Print and shaded views of the part. All mm, measured from the part's lowest x, y and z. A direction names the side the tool comes from. Coordinates: 2 decimals unless noted, no trailing zeros. Order: outer loops, then holes, each group sorted by start corner. A loop starts at its lowest first (then second) coordinate and runs counter-clockwise, first axis right, second up. Notation, with made-up numbers: M -7.75,-35 L 38.25,-35 A21 ccw 38.25,-20 Z; hole C 47,2 d2. An arc over 180 degrees is marked long. Use a Markdown table: item, result. Add a question column.
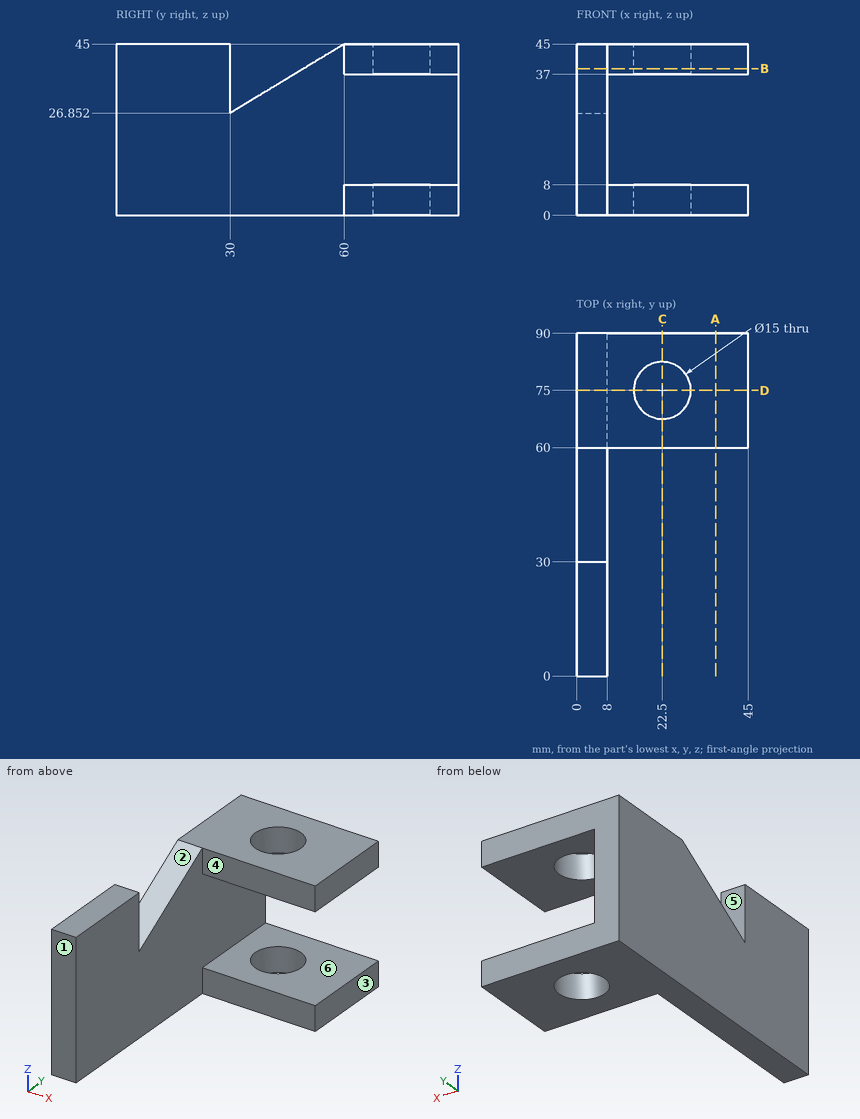
(1) Drop flat-ended pins along their axis: P1, Ø15, axis at x = 21, y = 74.5, coming from the -Z side; P2, Ø8, axis at x = 24.5, z = 15.5, coming from the -Y side; P3, Ø1, axis at y = 52, z = 19.5, coming from the +X side; P4, Ø6.5, axis at x = 34.5, z = 42, coming from the -Y side. Give the stop position or say it passes through.
(2) Drill centre lines: line 1 along Y through (x, z) = (22.5, 40.75); line 2 along Z through (x, y) = (33, 84); line 3 along Y through (x, z) = (39.5, 6). Where is each one in solid material? Low to high. Write a range as from..to.
(3) Mould opens along Y. For the marked faces 1, 2 and 3 say: released by +Y, released by -Y, zero draft, split by the parting line, or undercut.
(4) Slice it at C-C on x = 22.5. Give the cut face in (y, z).
(5) Which spindle directions (+Z, -Z, +X, -X, +Y, -Y) get a long thin tool onto all of the face, cutting with end or side? Do the marked faces 4, 5 and 6. Say none if no direction does.
(6) Slice it at A-A on x = 36.5. Give the cut face in (y, z).
(7) Slice it at B-B on z = 38.5. Give the cut face in (x, y) (3 decimals), and give its area (3 significant figures).
(8) Slice it at D-D on y = 75. Give the cut face in (x, z).
Solutions:
| question | item | result |
|---|---|---|
| 1 | P1 | z = 0 |
| 1 | P2 | through |
| 1 | P3 | x = 8 |
| 1 | P4 | y = 60 |
| 2 | line 1 | 60..67.5, 82.5..90 |
| 2 | line 2 | 0..8, 37..45 |
| 2 | line 3 | 60..90 |
| 3 | face 1 | released by -Y |
| 3 | face 2 | undercut |
| 3 | face 3 | zero draft |
| 4 | outline | M 60,0 L 67.5,0 L 67.5,8 L 60,8 Z; M 60,37 L 67.5,37 L 67.5,45 L 60,45 Z; M 82.5,0 L 90,0 L 90,8 L 82.5,8 Z; M 82.5,37 L 90,37 L 90,45 L 82.5,45 Z |
| 5 | face 4 | +Z, -Z, +X, -Y |
| 5 | face 5 | +Z, +X, -X |
| 5 | face 6 | +X, +Y, -Y |
| 6 | outline | M 60,0 L 90,0 L 90,8 L 60,8 Z; M 60,37 L 90,37 L 90,45 L 60,45 Z |
| 7 | outline | M 0,0 L 8,0 L 8,30 L 0,30 Z; M 0,49.255 L 8,49.255 L 8,60 L 45,60 L 45,90 L 0,90 Z; hole C 22.5,75 d15 |
| 7 | area | 1,500 mm² |
| 8 | outline | M 0,0 L 15,0 L 15,8 L 8,8 L 8,37 L 15,37 L 15,45 L 0,45 Z; M 30,0 L 45,0 L 45,8 L 30,8 Z; M 30,37 L 45,37 L 45,45 L 30,45 Z |
